```python
from build123d import *

# Parameters (mm, degrees)
SKETCH1_W               = 93
SKETCH1_H               = 130
SKETCH1_W_2             = 77
SKETCH1_H_2             = 114
BOSS_EXTRUDE1_DEPTH     = 22.5
CUT_EXTRUDE1_START      = 32
SKETCH2_R               = 11.1
CUT_EXTRUDE1_DEPTH      = 111.180343226
CUT_EXTRUDE2_START      = -45
SKETCH3_R               = 11.1
SKETCH3_R_2             = 18.75
CUT_EXTRUDE2_DEPTH      = 98.180343226
CUT_EXTRUDE3_DEPTH      = 143.180343226
CUT_EXTRUDE3_DEPTH_BACK = 143.180343226
SKETCH4_R               = 1.6
CUT_EXTRUDE4_START      = -45
SKETCH5_R               = 1.35
CUT_EXTRUDE4_DEPTH      = 98.180343226
CHAMFER1_SIZE           = 5
CUT_EXTRUDE5_DEPTH      = 143.180343226
CUT_EXTRUDE5_DEPTH_BACK = 143.180343226
SKETCH6_W               = 106
SKETCH6_H               = 10
CHAMFER2_SIZE           = 5
SKETCH11_W              = 25
SKETCH11_H              = 10
CUT_EXTRUDE7_DEPTH      = 134.098647626
FILLET2_R               = 3


with BuildPart() as part:
    # Sketch1 → Boss-Extrude1 (new, symmetric)
    with BuildSketch(Plane.XY):
        with Locations((-6.5, 65)):
            Rectangle(SKETCH1_W, SKETCH1_H)
        with Locations((-6.5, 65)):
            Rectangle(SKETCH1_W_2, SKETCH1_H_2, mode=Mode.SUBTRACT)
    extrude(amount=BOSS_EXTRUDE1_DEPTH, both=True)

    # Sketch2 → Cut-Extrude1 (cut, through all)
    with BuildSketch(Plane(origin=(0, 0, 0), x_dir=(0, 0, -1), z_dir=(1, 0, 0)).offset(CUT_EXTRUDE1_START)):
        with Locations(Location((0, 88.73, 0), (0, 0, 180))):
            Circle(SKETCH2_R)
        with Locations(Location((0, 30, 0), (0, 0, 180))):
            Circle(SKETCH2_R)
    extrude(amount=CUT_EXTRUDE1_DEPTH, mode=Mode.SUBTRACT)

    # Sketch3 → Cut-Extrude2 (cut, through all)
    with BuildSketch(Plane(origin=(0, 0, 0), x_dir=(0, 0, -1), z_dir=(1, 0, 0)).offset(CUT_EXTRUDE2_START)):
        with Locations(Location((0, 88.73, 0), (0, 0, 180))):
            Circle(SKETCH3_R)
        with Locations((0, 37)):
            Circle(SKETCH3_R_2)
    extrude(amount=-CUT_EXTRUDE2_DEPTH, mode=Mode.SUBTRACT)

    # Sketch4 → Cut-Extrude3 (cut, two sides: drawn at the far end of the back side and taken through both)
    with BuildSketch(Plane(origin=(0, 0, 0), x_dir=(1, 0, 0), z_dir=(0, 1, 0)).offset(-CUT_EXTRUDE3_DEPTH_BACK)):
        with Locations(Location((-12.5, 0, 0), (0, 0, 270))):
            Circle(SKETCH4_R)
        with Locations(Location((0, 12.5, 0), (0, 0, 270))):
            Circle(SKETCH4_R)
        with Locations(Location((12.5, 0, 0), (0, 0, 270))):
            Circle(SKETCH4_R)
        with Locations(Location((0, -12.5, 0), (0, 0, 270))):
            Circle(SKETCH4_R)
        with BuildLine():
            Line((-1.5875, 2.749630657), (1.5875, 2.749630657))
            ThreePointArc((1.5875, 2.749630657), (0, -3.175), (-1.5875, 2.749630657))
        make_face()
    extrude(amount=CUT_EXTRUDE3_DEPTH + CUT_EXTRUDE3_DEPTH_BACK, mode=Mode.SUBTRACT)

    # Sketch5 → Cut-Extrude4 (cut, through all)
    with BuildSketch(Plane(origin=(0, 0, 0), x_dir=(0, 0, -1), z_dir=(1, 0, 0)).offset(CUT_EXTRUDE4_START)):
        with Locations((18.589603123, 18.410396877)):
            Circle(SKETCH5_R)
        with Locations((-18.589603123, 18.410396877)):
            Circle(SKETCH5_R)
        with Locations((-18.589603123, 55.589603123)):
            Circle(SKETCH5_R)
        with Locations((18.589603123, 55.589603123)):
            Circle(SKETCH5_R)
    extrude(amount=-CUT_EXTRUDE4_DEPTH, mode=Mode.SUBTRACT)

    # Chamfer1
    chamfer1_edges = [part.edges().sort_by_distance(p)[0] for p in [
        (40, 65, 22.5),
        (40, 65, -22.5),
    ]]
    chamfer(chamfer1_edges, length=CHAMFER1_SIZE)

    # Sketch6 → Cut-Extrude5 (cut, two sides: drawn at the far end of the back side and taken through both)
    with BuildSketch(Plane.XY.offset(-CUT_EXTRUDE5_DEPTH_BACK)):
        with Locations((0, 125)):
            Rectangle(SKETCH6_W, SKETCH6_H)
    extrude(amount=CUT_EXTRUDE5_DEPTH + CUT_EXTRUDE5_DEPTH_BACK, mode=Mode.SUBTRACT)

    # Chamfer2
    chamfer2_edges = [part.edges().sort_by_distance(p)[0] for p in [
        (-45, 8, 0),
        (32, 8, 0),
    ]]
    chamfer(chamfer2_edges, length=CHAMFER2_SIZE)

    # Sketch11 → Cut-Extrude7 (cut, through all)
    with BuildSketch(Plane(origin=(0, 0, 0), x_dir=(0, 0, -1), z_dir=(1, 0, 0))):
        with Locations((0, 59.365)):
            Rectangle(SKETCH11_W, SKETCH11_H)
    extrude(amount=CUT_EXTRUDE7_DEPTH, mode=Mode.SUBTRACT)

    # Fillet2
    fillet2_edges = [part.edges().sort_by_distance(p)[0] for p in [
        (36, 54.365, -12.5),
        (36, 64.365, -12.5),
        (36, 64.365, 12.5),
        (36, 54.365, 12.5),
    ]]
    fillet(fillet2_edges, radius=FILLET2_R)


solid = part.part
```
CAD build for the part. Positions are in the model's coordinates, mm. A direction names the side the tool comes from. Give positions to 0.01 mm unless a question says otherwise; leave off trailing zeros. Write each loop counter-clockwise with the first axis right and the second up, starting at its lowest first coordinate (ties: lowest second). Pieces come first, ordered by that corner, then holes. Notation, with made-up numbers: M 48.25,-31.5 L 66.25,-31.5 A25 ccw 66.25,-3.5 Z; hole C 25.5,8 d5. An arc over 180 degrees is marked long. Return JSON: item names as keys, results as strings. Group by question number.
(1) Mould opens along X. For faces 1 (the face through (0.07, 3.94, 10.9)), 2 (the face through (35.94, 79.37, 5.97)), 3 (the face through (-13.92, 3.94, 0.74)), 4 (the face through (40, 46, 0)) say: pulls with the +X half, pulls with the -X half, needs draft (parallel to the pull), parting line crosses it, or undercut.
(2) Band-saw the part on C-C (x = 0). Give the cut face in (y, z) (3 decimals), and give its area (3 significant figures).
(3) Flat gauge pins, fed straight in: pin 1 Ø1.6 at (y, z) = (18.41, -18.59) entering from -X; pin 2 Ø20 at (y, z) = (30, 0) entering from -X; pin 3 Ø3 at (y, z) = (55.59, 18.59) entering from -X; pin 4 Ø1 at (x, z) = (-18, -2) entering from +Y. Where does each tip first touch, or does it go through?
(4) Band-saw the part on D-D (z = -4.5). State how many separate pieces and enclosed holes the cut face has, and give its area (3 significant figures).
(5) Band-saw the part on A-A (y = 88.73). Give the cut face in (x, z), and give its area (3 significant figures).
(6) 3-axis set-ups, long thin cutter, end or side, ignore diameter. For faces 5 (the face through (0, 4, -2.75)), 6 (the face through (37.5, 59.2, 20)), 7 (the face through (36.056, 63.463, -11.645)), 8 (the face through (-48.94, 54.27, 18.88)): which of +Z, -Z, +X, -X, +Y, -Y reach the whole face in a straight line?
(7) Drill centre lines: L1, parallel to Z at x = 0, y = 2 (3 decimals); L2, parallel to Z at x = -12.5, y = 6.25; L3, parallel to Z at x = 34, y = 88. Where is each one in solid material? Low to high. Write a range as [from, to].
(8) Band-saw the part on B-B (x = -12.5). Give the cut face in (y, z), and give its area (3 significant figures).
Entries:
{
 "1": {"face 1": "undercut", "face 2": "needs draft", "face 3": "undercut", "face 4": "pulls with the +X half"},
 "2": {"outline": "M 0,-22.5 L 8,-22.5 L 8,-14.1 L 0,-14.1 Z; M 0,-10.9 L 8,-10.9 L 8,-2.75 L 0,-2.75 Z; M 0,3.175 L 8,3.175 L 8,10.9 L 0,10.9 Z; M 0,14.1 L 8,14.1 L 8,22.5 L 0,22.5 Z", "area": "261 mm^2"},
 "3": {"pin 1": "stops at x = 32", "pin 2": "passes through", "pin 3": "stops at x = -53", "pin 4": "stops at y = 8"},
 "4": {"separate pieces": "6", "enclosed holes": "0", "area": "1,700 mm^2"},
 "5": {"outline": "M -53,-22.5 L -45,-22.5 L -45,-11.1 L -53,-11.1 Z; M -53,11.1 L -45,11.1 L -45,22.5 L -53,22.5 Z; M 32,-22.5 L 35,-22.5 L 40,-17.5 L 40,-11.1 L 32,-11.1 Z; M 32,11.1 L 40,11.1 L 40,17.5 L 35,22.5 L 32,22.5 Z", "area": "340 mm^2"},
 "6": {"face 5": "+Y, -Y", "face 6": "+Z, +X, +Y, -Y", "face 7": "+X", "face 8": "-X"},
 "7": {"L1": "z = [-22.5, -14.1], [-10.9, -2.75], [3.175, 10.9], [14.1, 22.5]", "L2": "z = [-22.5, -1.6], [1.6, 22.5]", "L3": "z = [-22.5, -11.08], [11.08, 22.5]"},
 "8": {"outline": "M 0,-22.5 L 8,-22.5 L 8,-1.6 L 0,-1.6 Z; M 0,1.6 L 8,1.6 L 8,22.5 L 0,22.5 Z", "area": "334 mm^2"}
}
